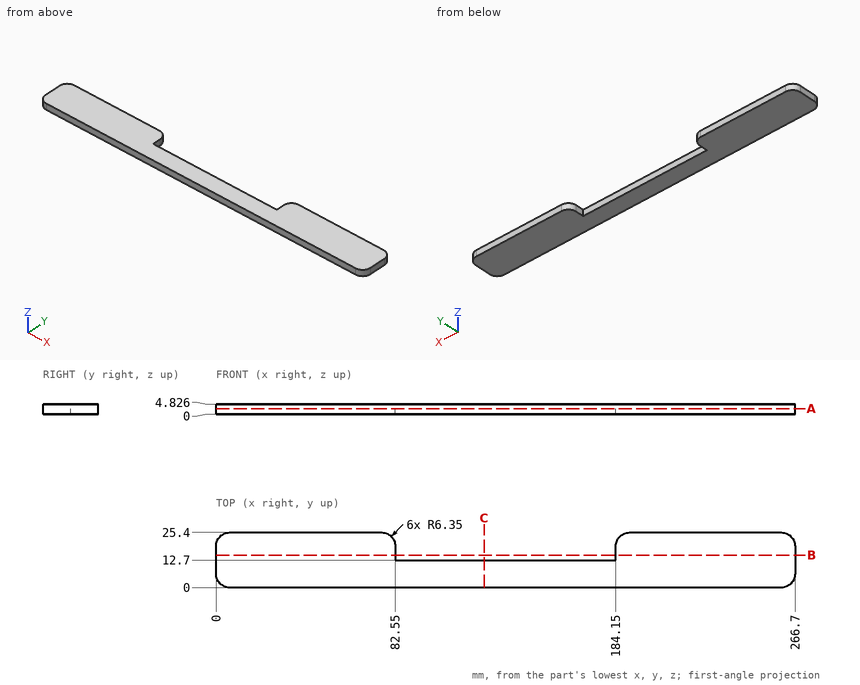
Answer from the drawing. Dimensions are ordinates in mm from the lowest x, y and z of the part. Give positions to 0.01 mm unless a question says otherwise; leave off trailing zeros. Loops run counter-clockwise (first coordinate to the right, second up) from the corner with the lowest first, then second, coordinate; pieces in that order, holes last. Notation, with made-up numbers: (10, 12) - (47, 12) arc R27 ccw to (47, 29) - close; hole circle Ø8 at (76, 37). An arc over 180 degrees is marked (long way). Write each question's results on one line, items separated by ' | '.
1. Find section C-C, the plane x = 123.5. Write down the section's boundary in (y, z).
Resolved:
outline: (0, 0) - (12.7, 0) - (12.7, 4.83) - (0, 4.83) - close
2. Find section B-B, the plane y = 15. Write down the section's boundary in (x, z), then the cut area to 3 significant figures.
Resolved:
outline: (0, 0) - (82.55, 0) - (82.55, 4.83) - (0, 4.83) - close; (184.15, 0) - (266.7, 0) - (266.7, 4.83) - (184.15, 4.83) - close | area: 797 mm^2
3. Consider probe 1 along X at (y, z) = (13, 2.7); probe 2 along Y at (x, z) = (166, 4.4). Determine where each line is inside the solid, lowest interval first. Write a range as from..to.
Resolved:
probe 1: x = 0..82.55, 184.15..266.7 | probe 2: y = 0..12.7
4. A flat-ended cylindrical pin translates along its axis: P1, Ø2, axis at x = 124.5, z = 1, coming from the +Y side. Find the tip coordinate at first contact, or state that the pin passes through.
Resolved:
P1: stops at y = 12.7
5. Find section A-A, the plane z = 2.65. Write down the section's boundary in (x, y), then the cut area to 3 significant figures.
Resolved:
outline: (0, 6.35) arc R6.35 ccw to (6.35, 0) - (260.35, 0) arc R6.35 ccw to (266.7, 6.35) - (266.7, 19.05) arc R6.35 ccw to (260.35, 25.4) - (190.5, 25.4) arc R6.35 ccw to (184.15, 19.05) - (184.15, 12.7) - (82.55, 12.7) - (82.55, 19.05) arc R6.35 ccw to (76.2, 25.4) - (6.35, 25.4) arc R6.35 ccw to (0, 19.05) - close | area: 5,430 mm^2
